Model file for the job. Use its own axes, mm. A direction names the side the tool comes from. Coordinates: 2 decimals unless noted, no trailing zeros. Write each loop counter-clockwise with the first axis right and the second up, starting at its lowest first coordinate (ties: lowest second). Pieces come first, ordered by that corner, then holes. Notation, with made-up numbers: M 64,8.25 L 112,8.25 A31 ccw 112,39.25 Z; hole C 69.5,50.25 d3. An arc over 180 degrees is marked long. One line per question, with ' | ' between items. Start each with the question number.
(1) Cut at A-A (z = -15). Write the cut outline in (x, y), plus the area to 4 significant figures.
(2) Cut at C-C (x = 4). Write the cut outline in (y, z), plus the area to 3 significant figures.
(3) Wall check: probe 1 along Y at (x, z) = (3.25, -9); probe 2 along Y at (x, z) = (2.5, -1.75); probe 3 along X at (y, z) = (10, -15.25). Give the ranges that are in metal, low to high.
(4) Tool access for faces 1 (the face through (2, 22, -15)), 2 (the face through (1, 15, -22.5)), 3 (the face through (1, 15, -7.5)): list every direction of +Z, -Z, +X, -X, +Y, -Y with a clear straight run to the whole face (end or side of a thin tool).
(5) Cut at D-D (x = 12.25). Write the cut outline in (y, z).
(6) Cut at B-B (y = 21). Write the cut outline in (x, z).
(7) Flat gauge pins, fed straight in: pin 1 Ø1.6 at (x, y) = (1.5, 16) entering from -Z; pin 2 Ø0.6 at (x, y) = (0.5, 12.5) entering from +Z; pin 3 Ø7.5 at (x, z) = (11, -12.5) entering from +Y; pin 4 Ø2 at (y, z) = (22, -24) entering from +X. Where does each tip first touch, or does it go through?
Autodesk Inventor part; units mm, degrees
ref_plane "YZ Plane" through (0, 0, 0) normal (1, 0, 0) x (0, 1, 0)
ref_plane "XZ Plane" through (0, 0, 0) normal (0, 1, 0) x (-1, 0, 0)
ref_plane "XY Plane" through (0, 0, 0) normal (0, 0, 1) x (1, 0, 0)
sketch "草圖1" plane through (0, 0, 0) normal (0, 1, 0) x (-1, 0, 0)
  line L0 (0, 0) -> (-15, 0)
  line L1 (-15, 0) -> (-15, -30)
  line L2 (-15, -30) -> (0, -30)
  line L3 (0, -30) -> (0, 0)
  dimension "d0" = 15
  dimension "d1" = 30
extrude "擠出1" add sketch "草圖1" along normal blind 5
fillet "圓角1" radius 2 4 edges at (15, 2.5, 0) (15, 2.5, -30) (0, 2.5, 0) (0, 2.5, -30)
sketch "草圖2" plane through (0, 5, 0) normal (0, 1, 0) x (1, 0, 0)
  line L0 (13, 30) -> (2, 30)
  line L1 (0, 28) -> (0, 2)
  line L2 (2, 30) -> (2, 15)
  arc A0 (2, 7.5) -> (2, 22.5) centre (2, 15) ccw
  line L3 (2, 15) -> (2, 7.5)
  line L4 (2, 15) -> (2, 22.5)
  line L5 (2, 22.5) -> (0, 22.5)
  line L6 (2, 7.5) -> (0, 7.5)
  line L7 (0, 22.5) -> (0, 7.5)
  point P0 (0, 0)
  dimension "d8" = 15
  dimension "d9" = 15
extrude "擠出3" add sketch "草圖2" along normal blind 15 contours A0 L3 L2
extrude "擠出4" add sketch "草圖2" along normal blind 20 contours L5 L2 L3 L6 L1
properties part number "孔1"
Filled in:
1) outline: M 0,0 L 15,0 L 15,5 L 9.5,5 L 9.5,20 L 2,20 L 2,25 L 0,25 Z | area: 227.5 mm²
2) outline: M 0,-30 L 5,-30 L 5,-22.23 L 20,-22.23 L 20,-7.77 L 5,-7.77 L 5,0 L 0,0 Z | area: 367 mm²
3) probe 1: 0 to 20 | probe 2: 0 to 5 | probe 3: 0 to 9.5
4) face 1: +Z, -Z, +X, +Y | face 2: -Z, +X, -X, +Y | face 3: +Z, +X, -X, +Y
5) outline: M 0,-30 L 5,-30 L 5,0 L 0,0 Z
6) outline: M 0,-22.5 L 2,-22.5 L 2,-7.5 L 0,-7.5 Z
7) pin 1: z = -22.5 | pin 2: z = -7.5 | pin 3: y = 20 | pin 4: through
